Read the model definition and answer for the solid it produces. Units are mm, in the model's axes. Face numbers are marked on the shaded views. Coordinates: 2 decimals unless noted, no trailing zeros. Order: outer loops, then holes, each group sorted by start corner. A loop starts at its lowest first (then second) coordinate and runs counter-clockwise, first axis right, second up.
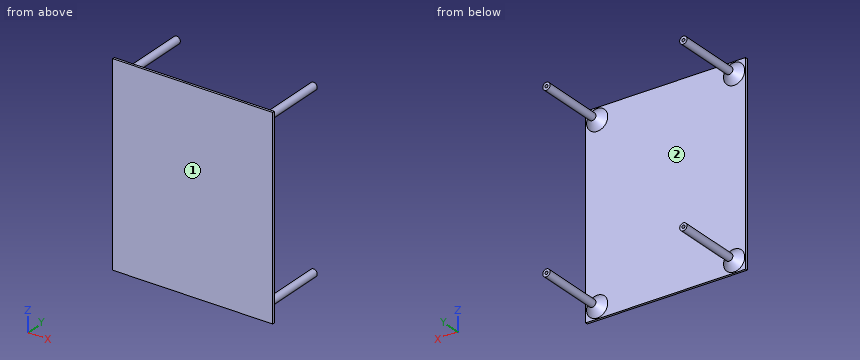
```python
from build123d import *

# Parameters (mm, degrees)
SKETCH_1_W          = 69.5
SKETCH_1_H          = 85
EXTRUDE_1_DEPTH     = 1
SKETCH_2_R          = 1.6
EXTRUDE_2_DEPTH     = 31
SKETCH_3_R          = 0.65
CUT_EXTRUDE_1_DEPTH = 5
CHAMFER_1_SIZE      = 3


with BuildPart() as part:
    # Эскиз1 → Бобышка-Вытянуть1 (new body)
    with BuildSketch(Plane(origin=(0, 0, 0), x_dir=(1, 0, 0), z_dir=(0, 1, 0))):
        with Locations((6.099344978, -9.693231441)):
            Rectangle(SKETCH_1_W, SKETCH_1_H)
    extrude(amount=EXTRUDE_1_DEPTH)

    # Эскиз2 → Бобышка-Вытянуть2 (add)
    with BuildSketch(Plane(origin=(0, 1, 0), x_dir=(1, 0, 0), z_dir=(0, 1, 0))):
        with Locations((-23.650655022, 27.806768559)):
            Circle(SKETCH_2_R)
        with Locations((35.849344978, 27.806768559)):
            Circle(SKETCH_2_R)
        with Locations((35.849344978, -47.193231441)):
            Circle(SKETCH_2_R)
        with Locations((-23.650655022, -47.193231441)):
            Circle(SKETCH_2_R)
    extrude(amount=EXTRUDE_2_DEPTH)

    # Эскиз3 → Вырез-Вытянуть1 (cut)
    with BuildSketch(Plane(origin=(0, 32, 0), x_dir=(1, 0, 0), z_dir=(0, 1, 0))):
        with Locations((-23.650655022, -47.193231441)):
            Circle(SKETCH_3_R)
        with Locations((35.849344978, -47.193231441)):
            Circle(SKETCH_3_R)
        with Locations((35.849344978, 27.806768559)):
            Circle(SKETCH_3_R)
        with Locations((-23.650655022, 27.806768559)):
            Circle(SKETCH_3_R)
    extrude(amount=-CUT_EXTRUDE_1_DEPTH, mode=Mode.SUBTRACT)

    # Фаска1
    chamfer_1_edges = [part.edges().sort_by_distance(p)[0] for p in [
        (-25.250655022, 1, -27.806768559),
        (34.249344978, 1, -27.806768559),
        (34.249344978, 1, 47.193231441),
        (-25.250655022, 1, 47.193231441),
    ]]
    chamfer(chamfer_1_edges, length=CHAMFER_1_SIZE)


solid = part.part
```
1) Determine the mould class of the marked faces 1 and 2 for opening direction Z: pulls with the +Z half, pulls with the -Z half, needs draft (parallel to the pull), parting line crosses it, or undercut.
A:
face 1: needs draft
face 2: undercut
2) A cutting plane is placed at D-D, the plane y = 18. Determine the outline of the cut face in (x, z), and give its area (3 significant figures).
A:
outline: circle Ø3.2 at (-23.65, -27.81); circle Ø3.2 at (-23.65, 47.19); circle Ø3.2 at (35.85, -27.81); circle Ø3.2 at (35.85, 47.19)
area: 32.2 mm2
3) A cutting plane is placed at C-C, the plane y = 2.5. Determine the outline of the cut face in (x, z).
A:
outline: circle Ø6.2 at (-23.65, -27.81); circle Ø6.2 at (-23.65, 47.19); circle Ø6.2 at (35.85, -27.81); circle Ø6.2 at (35.85, 47.19)
4) A cutting plane is placed at A-A, the plane x = -1.5. Determine the outline of the cut face in (y, z).
A:
outline: (0, -32.81) - (1, -32.81) - (1, 52.19) - (0, 52.19) - close
5) Flat-ended cylindrical pins translate along their axes: pin 1 Ø6 at (x, z) = (3.5, -22) entering from +Y; pin 2 Ø1.4 at (x, z) = (-23.5, -28) entering from +Y. Find the tip coordinate at first contact, or state that the pin passes through.
A:
pin 1: stops at y = 1
pin 2: stops at y = 32
6) A cutting plane is placed at B-B, the plane z = 1. Determine the outline of the cut face in (x, y), and give its area (3 significant figures).
A:
outline: (-28.65, 0) - (40.85, 0) - (40.85, 1) - (-28.65, 1) - close
area: 69.5 mm2
7) Straight lines are drawn through the part: line 1 (Y direction, x = 15, z = 20); line 2 (X direction, y = 14.5, z = 47.5); line 3 (X direction, y = 23.5, z = -28.5). For each, find the intervals that lie inside material, in ascending order.
A:
line 1: y = 0 to 1
line 2: x = -25.22 to -22.08, 34.28 to 37.42
line 3: x = -25.09 to -22.21, 34.41 to 37.29
